```python
from build123d import *

# Parameters (mm, degrees)
F0_W      = 8
F0_H      = 30
F0_W_2    = 3
F0_W_3    = 20.5
F0_H_2    = 10
F1_DEPTH  = 15
F2_DEPTH  = 2
F3_SIZE   = 2
F4_R      = 0.85
F5_DEPTH  = 15.001
F6_R      = 1
F6_R_2    = 7.5
F7_DEPTH  = 1.5
F8_W      = 3
F8_H      = 13
F9_DEPTH  = 2
F10_W     = 2
F10_H     = 13
F11_DEPTH = 2
F12_ANGLE = 90
F13_R     = 0.85
F14_DEPTH = 1.5
F15_W     = 33
F15_H     = 34
F16_DEPTH = 10
F17_W     = 20
F17_H     = 22
F17_R     = 0.85
F17_R_2   = 7.5
F18_DEPTH = 10
F19_R     = 0.85
F20_DEPTH = 10


with BuildPart() as f1:
    # F0 (on Top) → F1 (new body)
    with BuildSketch(Plane.XY):
        with Locations((-16.5, 0)):
            Rectangle(F0_W, F0_H)
        with Locations((-11, 0)):
            Rectangle(F0_W_2, F0_H)
        with Locations((-5.5, 0)):
            Rectangle(F0_W, F0_H)
        Polygon((1.5, 15), (-1.5, 15), (-1.5, -15), (0, -15), (1.5, -15), align=None)
        with Locations((5.5, 0)):
            Rectangle(F0_W, F0_H)
        with Locations((11, 0)):
            Rectangle(F0_W_2, F0_H)
        Polygon((9.5, -15), (1.5, -15), (0, -15), (0, -17), (20.5, -17), (20.5, -15), (12.5, -15), align=None)
        with Locations((16.5, 0)):
            Rectangle(F0_W, F0_H)
        with Locations((10.25, -22)):
            Rectangle(F0_W_3, F0_H_2)
    extrude(amount=-F1_DEPTH)

    # F0 (on Top) → F2 (cut)
    with BuildSketch(Plane.XY):
        with Locations((-11, 0)):
            Rectangle(F0_W_2, F0_H)
        Polygon((1.5, 15), (-1.5, 15), (-1.5, -15), (0, -15), (1.5, -15), align=None)
        with Locations((11, 0)):
            Rectangle(F0_W_2, F0_H)
        Polygon((9.5, -15), (1.5, -15), (0, -15), (0, -17), (20.5, -17), (20.5, -15), (12.5, -15), align=None)
    extrude(amount=-F2_DEPTH, mode=Mode.SUBTRACT)

    # F3
    f3_edges = [f1.edges().sort_by_distance(p)[0] for p in [
        (-16.5, 15, 0),
        (-20.5, 0, 0),
        (20.5, 0, 0),
        (16.5, 15, 0),
        (5.5, 15, 0),
        (-5.5, 15, 0),
        (10.25, -27, 0),
        (20.5, -22, 0),
        (0, -22, 0),
    ]]
    chamfer(f3_edges, length=F3_SIZE)

    # F4 (on face) → F5 (cut, through all)
    with BuildSketch(Plane.XY):
        with Locations((-7.5, 7.5)):
            Circle(F4_R)
        with Locations((7.5, 7.5)):
            Circle(F4_R)
        with Locations((7.5, -7.5)):
            Circle(F4_R)
        with Locations((-7.5, -7.5)):
            Circle(F4_R)
    extrude(amount=-F5_DEPTH, mode=Mode.SUBTRACT)

    # F8 (on face) → F9 (cut)
    with BuildSketch(Plane(origin=(0, 15, 0), x_dir=(-1, 0, 0), z_dir=(0, 1, 0))):
        with Locations((11, -8.5)):
            Rectangle(F8_W, F8_H)
        Polygon((1.5, -15), (1.5, -2), (0, -2), (-1.5, -2), (-1.5, -15), (0, -15), align=None)
        with Locations((-11, -8.5)):
            Rectangle(F8_W, F8_H)
    extrude(amount=-F9_DEPTH, mode=Mode.SUBTRACT)

    # F10 (on face) → F11 (cut)
    with BuildSketch(Plane.YZ.offset(20.5)):
        with Locations((-16, -8.5)):
            Rectangle(F10_W, F10_H)
    extrude(amount=-F11_DEPTH, mode=Mode.SUBTRACT)

    # F15 (on face) → F16 (cut)
    with BuildSketch(Plane(origin=(0, 0, -15), x_dir=(1, 0, 0), z_dir=(0, 0, -1))):
        with Locations((0, 6)):
            Rectangle(F15_W, F15_H)
    extrude(amount=-F16_DEPTH, mode=Mode.SUBTRACT)



with BuildPart() as f7:
    # F6 (on face) → F7 (new body)
    with BuildSketch(Plane(origin=(0, 0, -15), x_dir=(1, 0, 0), z_dir=(0, 0, -1))):
        with BuildLine():
            ThreePointArc((10, 14.5), (9.5606601718, 15.5606601718), (8.5, 16))
            Line((8.5, 16), (-8.5, 16))
            ThreePointArc((-8.5, 16), (-9.5606601718, 15.5606601718), (-10, 14.5))
            Line((-10, 14.5), (-10, -14.5))
            ThreePointArc((-10, -14.5), (-9.5606601718, -15.5606601718), (-8.5, -16))
            Line((-8.5, -16), (8.5, -16))
            ThreePointArc((8.5, -16), (9.5606601718, -15.5606601718), (10, -14.5))
            Line((10, -14.5), (10, 14.5))
        make_face()
        with Locations((-7.5, -13.5)):
            Circle(F6_R, mode=Mode.SUBTRACT)
        with Locations((0, -13.5)):
            Circle(F6_R, mode=Mode.SUBTRACT)
        with Locations((7.5, -13.5)):
            Circle(F6_R, mode=Mode.SUBTRACT)
        with Locations((-7.5, 13.5)):
            Circle(F6_R, mode=Mode.SUBTRACT)
        Circle(F6_R_2, mode=Mode.SUBTRACT)
        with Locations((0, 13.5)):
            Circle(F6_R, mode=Mode.SUBTRACT)
        with Locations((7.5, 13.5)):
            Circle(F6_R, mode=Mode.SUBTRACT)
    extrude(amount=F7_DEPTH)


with BuildPart() as f7_1:
    # F12: moved
    add(f7.part.rotate(Axis((0, 0, -15), (0, 0, -1)), F12_ANGLE))

    # F13 (on face) → F14 (cut, through all)
    with BuildSketch(Plane(origin=(0, 0, -16.5), x_dir=(1, 0, 0), z_dir=(0, 0, -1))):
        with Locations((-7.5, -7.5)):
            Circle(F13_R)
        with Locations((7.5, -7.5)):
            Circle(F13_R)
        with Locations((-7.5, 7.5)):
            Circle(F13_R)
        with Locations((7.5, 7.5)):
            Circle(F13_R)
    extrude(amount=-F14_DEPTH, mode=Mode.SUBTRACT)


with BuildPart() as f18:
    # F17 (on face) → F18 (new body, through all)
    with BuildSketch(Plane(origin=(0, 0, -5), x_dir=(1, 0, 0), z_dir=(0, 0, -1))):
        Rectangle(F17_W, F17_H)
        with Locations((-7.5, -7.5)):
            Circle(F17_R, mode=Mode.SUBTRACT)
        with Locations((7.5, -7.5)):
            Circle(F17_R, mode=Mode.SUBTRACT)
        with Locations((-7.5, 7.5)):
            Circle(F17_R, mode=Mode.SUBTRACT)
        Circle(F17_R_2, mode=Mode.SUBTRACT)
        with Locations((7.5, 7.5)):
            Circle(F17_R, mode=Mode.SUBTRACT)
    extrude(amount=F18_DEPTH)


with BuildPart() as f1_1:
    add(f1.part)

    add(f18.part)  # F20 merges F18
    # F19 (on face) → F20 (join)
    with BuildSketch(Plane.XY):
        with Locations((7.5, 7.5)):
            Circle(F19_R)
        with Locations((-7.5, 7.5)):
            Circle(F19_R)
        with Locations((-7.5, -7.5)):
            Circle(F19_R)
        with Locations((7.5, -7.5)):
            Circle(F19_R)
    extrude(amount=-F20_DEPTH)


with BuildPart() as f22_1:
    # F22: instance of F1
    add(f1_1.part.mirror(Plane.YZ.offset(-30)))


solid = f22_1.part
```
The model under review builds one solid part; all positions refer to its coordinate system, in mm. A direction names the side the tool comes from. Round coordinates to 2 decimals unless told otherwise and drop trailing zeros. Write each loop counter-clockwise with the first axis right and the second up, starting at its lowest first coordinate (ties: lowest second). Pieces come first, ordered by that corner, then holes.
(1) Mouldability with a two-part tool opening along X and no side actions: class faces 4 (the flat face through (-60, 13, -8)), 5 (the flat face through (-79.5, -22.1, -1)), 6 (the flat face through (-75, -1, 0)) as +X half, -X half, draft (parallel to the pull), parting line (faces both ways), or undercut.
(2) We need section C-C on x = -55.5. Give the boundary of the cut face in (y, z), and give its area (3 significant figures).
(3) We need section B-B on y = -10. Give the boundary of the cut face in (x, z), and give its area (3 significant figures).
(4) Machinability: for faces 1 (the cylindrical face through (-67.957, 6.783, -12.465)), 2 (the flat face through (-78.5, -16, -8)), 3 (the flat face through (-47, 11, -10)), which of the approach directions +Z, -Z, +X, -X, +Y, -Y give a long, thin tool a straight path to every point of the face, cutting with its end or side? Answer none if there is none.
(5) Wall thickness on L1, parallel to X at y = -12, z = -5.75; L2, parallel to Y at x = -60.5, z = -8.5; L3, parallel to Z at x = -73, y = 10: over which ranges is each line inside the solid? List them lowest first.
(6) Insertion check: pin 1 (1.5 mm diameter, centred on x = -60.5, y = -19.5, fed in from +Z); pin 2 (0.5 mm diameter, centred on x = -67.5, y = 7.5, fed in from -Z); pin 3 (1.5 mm diameter, centred on x = -54, z = -12.5, fed in from -Y). Each pin has a flat end and moves straight along its axis. Give the tip position at first contact, or say it passes through.
Findings below:
1. face 4: undercut
1. face 5: -X half
1. face 6: draft
2. outline: (-15, -5) - (-11, -5) - (-11, -15) - (-6, -15) - (-6, -5) - (6, -5) - (6, -15) - (15, -15) - (15, -2) - (13, 0) - (-15, 0) - close
2. area: 288 mm2
3. outline: (-80.5, -15) - (-76.5, -15) - (-76.5, -5) - (-70, -5) - (-70, -15) - (-50, -15) - (-50, -5) - (-43.5, -5) - (-43.5, -15) - (-39.5, -15) - (-39.5, -2) - (-41.5, 0) - (-47.5, 0) - (-47.5, -2) - (-50.5, -2) - (-50.5, 0) - (-58.5, 0) - (-58.5, -2) - (-61.5, -2) - (-61.5, 0) - (-69.5, 0) - (-69.5, -2) - (-72.5, -2) - (-72.5, 0) - (-78.5, 0) - (-80.5, -2) - close
3. area: 463 mm2
4. face 1: -Z
4. face 2: +Z, -Z, -X
4. face 3: -Z, -Y
5. L1: x = -80.5 to -76.5, -43.5 to -39.5
5. L2: y = -27 to -23, -11 to -7.48, 7.48 to 13
5. L3: z = -5 to 0
6. pin 1: stops at z = -0.75
6. pin 2: stops at z = -10
6. pin 3: stops at y = -11
